Autodesk Inventor part; units mm, degrees
ref_plane "YZ Plane" through (0, 0, 0) normal (1, 0, 0) x (0, 1, 0)
ref_plane "XZ Plane" through (0, 0, 0) normal (0, 1, 0) x (-1, 0, 0)
ref_plane "XY Plane" through (0, 0, 0) normal (0, 0, 1) x (1, 0, 0)
sketch "Sketch1" plane through (0, 0, 0) normal (0, 1, 0) x (-1, 0, 0)
  circle A0 centre (0, 0) radius 3.5
  line L0 (1, -3.3541) -> (-1, -3.3541) construction
  line L1 (-1, -3.3541) -> (-1, -8.3541)
  line L2 (-1, -8.3541) -> (1, -8.3541)
  line L3 (1, -8.3541) -> (1, -3.3541)
  line L4 (0, 0) -> (0, 3.5) construction
  line L5 (8.3541, 1) -> (3.3541, 1)
  line L6 (8.3541, -1) -> (8.3541, 1)
  line L7 (3.3541, -1) -> (8.3541, -1)
  line L8 (-1, 8.3541) -> (-1, 3.3541)
  line L9 (1, 8.3541) -> (-1, 8.3541)
  line L10 (1, 3.3541) -> (1, 8.3541)
  line L11 (-8.3541, -1) -> (-3.3541, -1)
  line L12 (-8.3541, 1) -> (-8.3541, -1)
  line L13 (-3.3541, 1) -> (-8.3541, 1)
  line L14 (3.3541, -1) -> (1, -3.3541) construction
  line L15 (8.3541, -1) -> (1, -8.3541) construction
  dimension "d0" = 7
  dimension "d1" = 2
  dimension "d2" = 5
  dimension "d5" = 360
  dimension "d7" = 3.3292
  dimension "d8" = 10.4003
  dimension "d9" = 3.5355
extrude "Extrusion1" add sketch "Sketch1" along normal blind 5
sketch "Sketch2" plane through (0, 5, 0) normal (0, 1, 0) x (1, 0, 0)
  circle A0 centre (0, 0) radius 2.6
  line L0 (-1.6, -2.0494) -> (-1.6, 2.0494)
  line L1 (1.6, -2.0494) -> (1.6, 2.0494)
  line L2 (0, 0) -> (0, 2.6) construction
  dimension "d12" = 5.2
  dimension "d13" = 3.2
extrude "Extrusion2" cut sketch "Sketch2" against normal blind 3 contours L1 A0 L0
sketch "Sketch3" plane through (0, 5, 0) normal (0, 1, 0) x (1, 0, 0)
  line L0 (-1.6, -2.0494) -> (-1.6, 2.0494)
  arc A0 (1.6, 2.0494) -> (-1.6, 2.0494) centre (0, 0) ccw
  line L1 (1.6, 2.0494) -> (1.6, -2.0494)
  arc A1 (-1.6, -2.0494) -> (1.6, -2.0494) centre (0, 0) ccw
  arc A2 (-1, 3.3541) -> (-3.3541, 1) centre (0, 0) ccw
  line L2 (-3.3541, 1) -> (-8.3541, 1)
  line L3 (-8.3541, 1) -> (-8.3541, -1)
  line L4 (-8.3541, -1) -> (-3.3541, -1)
  arc A3 (-3.3541, -1) -> (-1, -3.3541) centre (0, 0) ccw
  line L5 (-1, -3.3541) -> (-1, -8.3541)
  line L6 (-1, -8.3541) -> (1, -8.3541)
  line L7 (1, -8.3541) -> (1, -3.3541)
  arc A4 (1, -3.3541) -> (3.3541, -1) centre (0, 0) ccw
  line L8 (3.3541, -1) -> (8.3541, -1)
  line L9 (8.3541, -1) -> (8.3541, 1)
  line L10 (8.3541, 1) -> (3.3541, 1)
  arc A5 (3.3541, 1) -> (1, 3.3541) centre (0, 0) ccw
  line L11 (1, 3.3541) -> (1, 8.3541)
  line L12 (1, 8.3541) -> (-1, 8.3541)
  line L13 (-1, 8.3541) -> (-1, 3.3541)
ref_plane "Work Plane1" through (2.25, 8, 0) normal (0, -1, 0) x (-1, 0, 0)
extrude "Extrusion3" add sketch "Sketch3" along normal up to surface (3 mm away)
properties part number "paddle rotor"
Geometry: final body of the model. Coordinates: model frame, mm. A direction names the side the tool comes from. Coordinates: 2 decimals unless noted, no trailing zeros. Loops run counter-clockwise (first coordinate to the right, second up) from the corner with the lowest first, then second, coordinate; pieces in that order, holes last. Notation, with made-up numbers: M -37,27 L 15,27 A22 ccw 15,59 Z; hole C 8,-26 d7. An arc over 180 degrees is marked long. One line per item, written item: value. Start each with the question number.
1) Cut plane B-B (z = -0.5). Return loops of the section in (x, y).
2) Cut plane A-A (y = 6.5). Return loops of the section in (x, z).
3) Reachability of faces 4 (the flat face through (-6, 4, 1)), 5 (the flat face through (1, 4, 6)), 6 (the flat face through (1, 4, -6)), 7 (the flat face through (-1, 4, -6)), 8 (the flat face through (0, 2, 0)) from +Z, -Z, +X, -X, +Y, -Y: full face, straight path, thin tool, end or side. Return the list, or none.
4) Cut plane D-D (x = 6.75). Return loops of the section in (y, z).
5) Material intervals for L1, parallel to X at y = 6, z = -3.75; L2, parallel to Y at x = -1.25, z = -1.5, sorted ascending. Write a range as from..to.
6) Cut plane C-C (y = 1.75). Return loops of the section in (x, z).
7) Pin query (flat end, axial travel): P1, Ø2.5, axis at y = 5.5, z = 5, coming from the +X side; P2, Ø4, axis at x = 6, y = 3, coming from the -Z side; P3, Ø2, axis at x = -3.5, y = 5, coming from the +Z side; P4, Ø2, axis at x = -6.5, z = -0.5, coming from the -Y side. Return the tip coordinate at first contact, or that it passes through.
8) Draft query along Z for faces 1 (the flat face through (-1.6, 5, 0)), 2 (the flat face through (-6, 4, -1)), 3 (the flat face through (-1, 4, 6)). Return one class per face: released by +Z, released by -Z, zero draft, split by the parting line, or undercut.
Evaluation:
1. outline: M -8.35,0 L 8.35,0 L 8.35,8 L 1.6,8 L 1.6,2 L -1.6,2 L -1.6,8 L -8.35,8 Z
2. outline: M -8.35,-1 L -3.35,-1 A3.5 ccw -1,-3.35 L -1,-8.35 L 1,-8.35 L 1,-3.35 A3.5 ccw 3.35,-1 L 8.35,-1 L 8.35,1 L 3.35,1 A3.5 ccw 1,3.35 L 1,8.35 L -1,8.35 L -1,3.35 A3.5 ccw -3.35,1 L -8.35,1 Z; hole M -1.6,-2.05 A2.6 ccw 1.6,-2.05 L 1.6,2.05 A2.6 ccw -1.6,2.05 Z
3. face 4: +Z, -X, +Y, -Y
3. face 5: +Z, +X, +Y, -Y
3. face 6: -Z, +X, +Y, -Y
3. face 7: -Z, -X, +Y, -Y
3. face 8: +Y
4. outline: M 0,-1 L 8,-1 L 8,1 L 0,1 Z
5. L1: -1..1
5. L2: 0..2
6. outline: M -8.35,-1 L -3.35,-1 A3.5 ccw -1,-3.35 L -1,-8.35 L 1,-8.35 L 1,-3.35 A3.5 ccw 3.35,-1 L 8.35,-1 L 8.35,1 L 3.35,1 A3.5 ccw 1,3.35 L 1,8.35 L -1,8.35 L -1,3.35 A3.5 ccw -3.35,1 L -8.35,1 Z
7. P1: x = 1
7. P2: z = -1
7. P3: z = 2.45
7. P4: y = 0
8. face 1: undercut
8. face 2: released by -Z
8. face 3: zero draft
